```python
from build123d import *

# Parameters (mm, degrees)
SKETCH1_W           = 300
SKETCH1_H           = 300
BOSS_EXTRUDE1_DEPTH = 5
SKETCH2_W           = 29
SKETCH2_H           = 59
CUT_EXTRUDE1_DEPTH  = 5
SKETCH3_W           = 5
SKETCH3_H           = 20
CUT_EXTRUDE2_DEPTH  = 5


with BuildPart() as part:
    # Sketch1 → Boss-Extrude1 (new body)
    with BuildSketch(Plane(origin=(0, 0, 0), x_dir=(1, 0, 0), z_dir=(0, 1, 0))):
        with Locations((150, 150)):
            Rectangle(SKETCH1_W, SKETCH1_H)
    extrude(amount=BOSS_EXTRUDE1_DEPTH)

    # Sketch2 → Cut-Extrude1 (cut)
    with BuildSketch(Plane(origin=(0, 5, 0), x_dir=(1, 0, 0), z_dir=(0, 1, 0))):
        with Locations((235.5, 125.25)):
            Rectangle(SKETCH2_W, SKETCH2_H)
        with Locations((64.5, 125.25)):
            Rectangle(SKETCH2_W, SKETCH2_H)
    extrude(amount=-CUT_EXTRUDE1_DEPTH, mode=Mode.SUBTRACT)

    # Sketch3 → Cut-Extrude2 (cut)
    with BuildSketch(Plane(origin=(0, 5, 0), x_dir=(1, 0, 0), z_dir=(0, 1, 0))):
        with Locations((267.5, 30)):
            Rectangle(SKETCH3_W, SKETCH3_H)
        with Locations((267.5, 150)):
            Rectangle(SKETCH3_W, SKETCH3_H)
        with Locations((267.5, 270)):
            Rectangle(SKETCH3_W, SKETCH3_H)
        with Locations((32.5, 30)):
            Rectangle(SKETCH3_W, SKETCH3_H)
        with Locations((32.5, 150)):
            Rectangle(SKETCH3_W, SKETCH3_H)
        with Locations((32.5, 270)):
            Rectangle(SKETCH3_W, SKETCH3_H)
    extrude(amount=-CUT_EXTRUDE2_DEPTH, mode=Mode.SUBTRACT)


solid = part.part
```
Work out the finished part from the listing and answer in its coordinate system (mm). Give positions to 0.01 mm unless a question says otherwise; leave off trailing zeros. Order: outer loops, then holes, each group sorted by start corner. A loop starts at its lowest first (then second) coordinate and runs counter-clockwise, first axis right, second up.
1. Straight lines are drawn through the part: L1, parallel to X at y = 3.25, z = -277; L2, parallel to X at y = 0.8, z = -149.5; L3, parallel to Z at x = 70.5, y = 1.35. For each, find the intervals that lie inside material, in ascending order.
Result sheet:
L1: x = 0 to 30, 35 to 265, 270 to 300
L2: x = 0 to 30, 35 to 50, 79 to 221, 250 to 265, 270 to 300
L3: z = -300 to -154.75, -95.75 to 0
2. Section A-A, the plane z = -120 is taken. Determine the outline of the cut face in (x, y).
Result sheet:
outline: (0, 0) - (50, 0) - (50, 5) - (0, 5) - close; (79, 0) - (221, 0) - (221, 5) - (79, 5) - close; (250, 0) - (300, 0) - (300, 5) - (250, 5) - close
3. Section B-B, the plane y = 3.45 is taken. Give the number of separate pieces and of enclosed holes in the cut face, and give its area (3 significant figures).
Result sheet:
separate pieces: 1
enclosed holes: 8
area: 86,000 mm2
